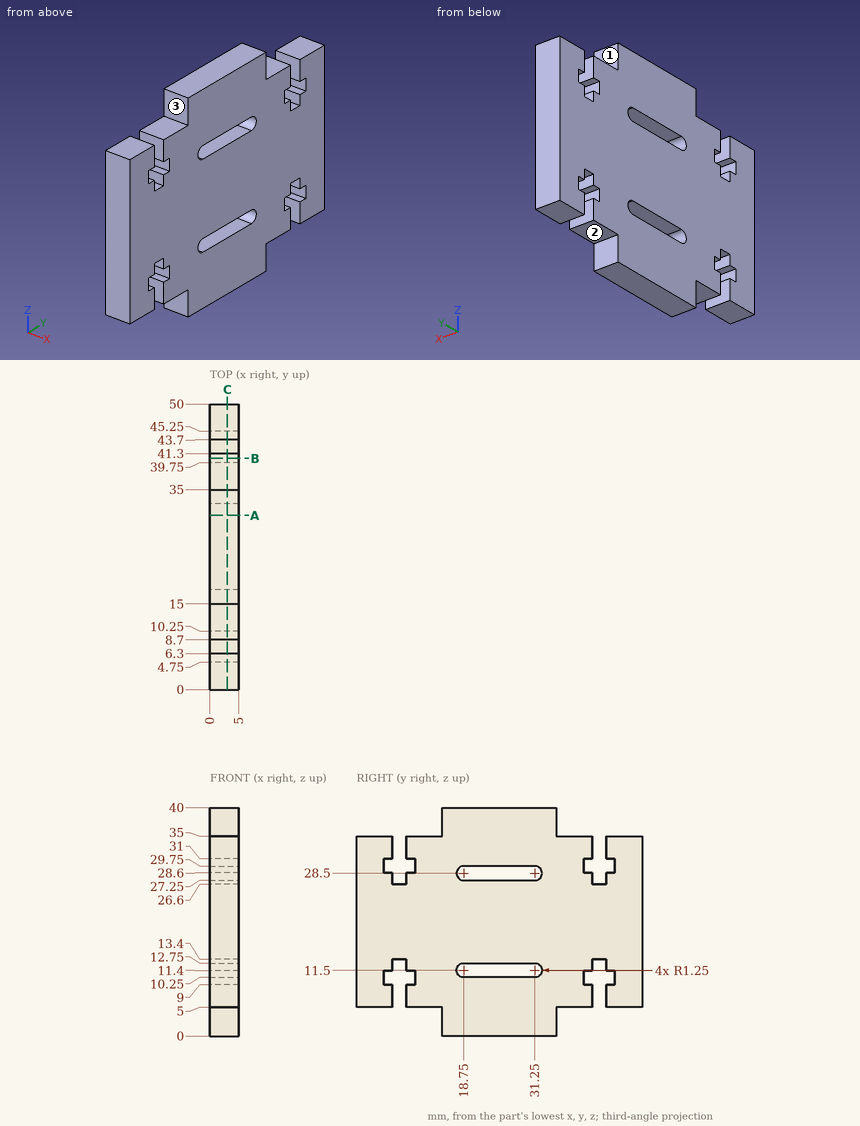
For this review, use the dimensioned drawing (mm, ordinates from the lowest corner) and the shaded views. A direction names the side the tool comes from. Give positions to 0.01 mm unless a question says otherwise; leave off trailing zeros. Write each loop counter-clockwise with the first axis right and the second up, starting at its lowest first coordinate (ties: lowest second). Pieces come first, ordered by that corner, then holes. Notation, with made-up numbers: M -19,25.5 L 30,25.5 A30 cw 30,53.5 Z; hole C 81,72 d3. An arc over 180 degrees is marked long. Answer as a JSON object with one key per item and string values. Group by question number.
Item 1: Consider section B-B on y = 40.5. Write out the cut boundary in (x, z), plus the area to 3 significant figures.
Item 2: Consider section A-A on y = 30.5. Write out the cut boundary in (x, z).
Item 3: Tool access review of the marked faces 1, 2 and 3: name each direction out of +Z, -Z, +X, -X, +Y, -Y from which nothing blocks a thin tool from reaching the whole face with its end or side.
Item 4: For probe 1 along Z at (x, y) = (3.9, 40); probe 2 along Z at (x, y) = (2.35, 23); probe 3 along Y at (x, z) = (1.75, 11), list the stretches that pass through material, from the lowest coordinate up. Write a range as [from, to].
Item 5: Consider section C-C on x = 3.05. Count the separate pieces of the cut face and the enclosed holes in it, plus the area to 3 significant figures.
Item 6: For pin 1 Ø0.8 at (x, y) = (2, 44.5) entering from +Z; pin 2 Ø1.5 at (x, z) = (3.5, 38) entering from +Y, all flat-tipped, find the tip position at first contact; note any pin that passes through.
Check result:
{
 "1": {"outline": "M 0,5 L 5,5 L 5,9 L 0,9 Z; M 0,11.4 L 5,11.4 L 5,28.6 L 0,28.6 Z; M 0,31 L 5,31 L 5,35 L 0,35 Z", "area": "126 mm^2"},
 "2": {"outline": "M 0,0 L 5,0 L 5,10.25 L 0,10.25 Z; M 0,12.75 L 5,12.75 L 5,27.25 L 0,27.25 Z; M 0,29.75 L 5,29.75 L 5,40 L 0,40 Z"},
 "3": {"face 1": "+Z, +X, -X, +Y", "face 2": "-Z, +X, -X, +Y", "face 3": "+Z, +X, -X, -Y"},
 "4": {"probe 1": "z = [5, 9], [11.4, 28.6], [31, 35]", "probe 2": "z = [0, 10.25], [12.75, 27.25], [29.75, 40]", "probe 3": "y = [0, 4.75], [10.25, 17.6], [32.4, 39.75], [45.25, 50]"},
 "5": {"separate pieces": "1", "enclosed holes": "2", "area": "1,520 mm^2"},
 "6": {"pin 1": "stops at z = 35", "pin 2": "stops at y = 35"}
}
